Verification items for this drawing (mm, ordinates from the low corner). Round coordinates to 2 decimals unless told otherwise and drop trailing zeros. Loops run counter-clockwise (first coordinate to the right, second up) from the corner with the lowest first, then second, coordinate; pieces in that order, holes last. Notation, with made-up numbers: M 63.25,70 L 107.25,70 A7 cw 107.25,76 Z; hole C 87,89 d11. An arc over 180 degrees is marked long. One line per item, written item: value.
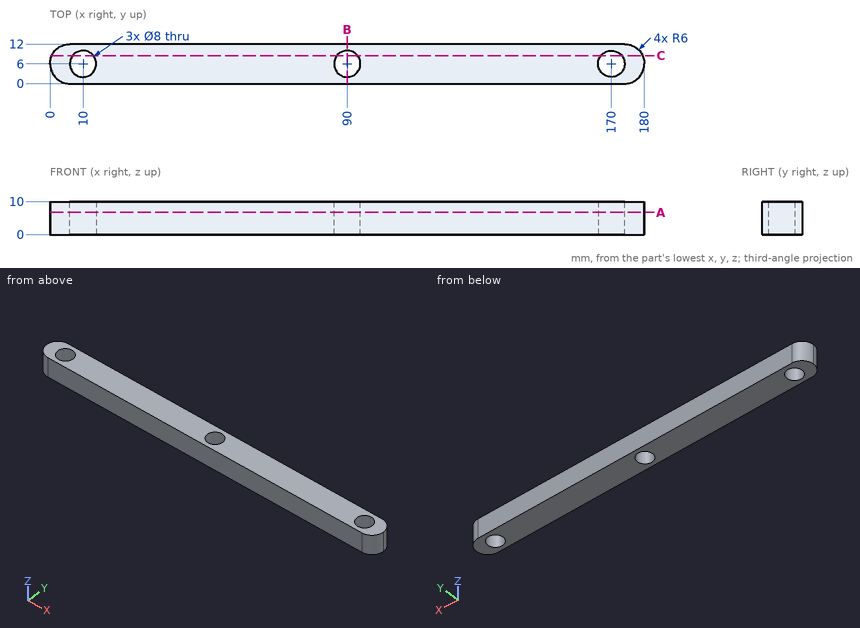
(1) Sectioned sample at A-A on z = 6.75. Count the separate pieces of the cut face and the enclosed holes in it, and give its area (3 significant figures).
Completed:
separate pieces: 1
enclosed holes: 3
area: 1,980 mm^2
(2) Sectioned sample at B-B on x = 90. Enter the section's corners in (y, z).
Completed:
outline: M 0,0 L 2,0 L 2,10 L 0,10 Z; M 10,0 L 12,0 L 12,10 L 10,10 Z
(3) Depth check by flat-ended pin: pin 1 Ø5 at (y, z) = (2.5, 2.5) entering from -X; pin 2 Ø3 at (y, z) = (4, 2.5) entering from +X. Enter the tip coordinate at first touch or a pass-through.
Completed:
pin 1: stops at x = 0.08
pin 2: stops at x = 179.98
(4) Thickness scan on L1, parallel to X at y = 6.5, z = 2; L2, parallel to Y at x = 10, z = 6; L3, parallel to X at y = 2.5, z = 4 (1 decimal). Record the ranges inside material, lowest first. Write a range as from..to.
Completed:
L1: x = 0.02..6.03, 13.97..86.03, 93.97..166.03, 173.97..179.98
L2: y = 0..2, 10..12
L3: x = 1.1..8.1, 11.9..88.1, 91.9..168.1, 171.9..178.9
(5) Sectioned sample at C-C on y = 8.5. Enter the section's corners in (x, z) (1 decimal).
Completed:
outline: M 0.5,0 L 6.9,0 L 6.9,10 L 0.5,10 Z; M 13.1,0 L 86.9,0 L 86.9,10 L 13.1,10 Z; M 93.1,0 L 166.9,0 L 166.9,10 L 93.1,10 Z; M 173.1,0 L 179.5,0 L 179.5,10 L 173.1,10 Z
